Check sheet for the drawn part. Datum: minimum x, y, z corner. Units: mm. Round coordinates to 2 decimals unless told otherwise and drop trailing zeros. Write each loop counter-clockwise with the first axis right and the second up, starting at its lowest first coordinate (ties: lowest second). Pieces come first, ordered by that corner, then holes. Notation, with made-up numbers: (74, 37) -> (103, 37) arc R20 cw to (103, 44) -> close; hole circle Ø4 at (26, -25.5). An arc over 180 degrees is marked (long way). One line per item, written item: value.
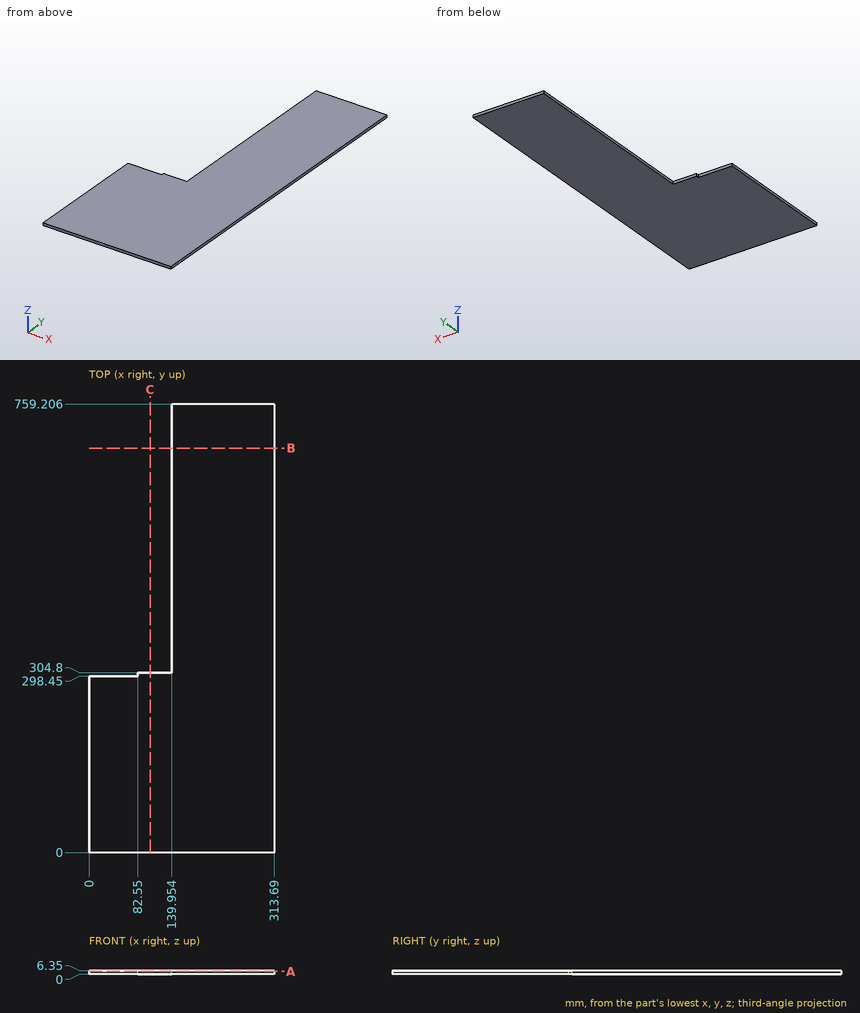
Item 1: Sectioned sample at A-A on z = 5. Enter the section's corners in (x, y).
Answer:
outline: (0, 0) -> (313.69, 0) -> (313.69, 759.21) -> (139.95, 759.21) -> (139.95, 304.8) -> (82.55, 304.8) -> (82.55, 298.45) -> (0, 298.45) -> close
Item 2: Thickness scan on line 1 (Y direction, x = 110, z = 1.75); line 2 (X direction, y = 433.5, z = 4); line 3 (Y direction, x = 17, z = 4.5). Record the ranges inside material, lowest first.
Answer:
line 1: y = 0 to 304.8
line 2: x = 139.95 to 313.69
line 3: y = 0 to 298.45
Item 3: Depth check by flat-ended pin: P1, Ø3, axis at x = 39, z = 4, coming from the +Y side; P2, Ø1.9, axis at x = 100.5, z = 3.5, coming from the +Y side; P3, Ø1.9, axis at y = 645, z = 3, coming from the -X side. Enter the tip coordinate at first touch or a pass-through.
Answer:
P1: stops at y = 298.45
P2: stops at y = 304.8
P3: stops at x = 139.95
Item 4: Sectioned sample at B-B on y = 684.5. Enter the section's corners in (x, z).
Answer:
outline: (139.95, 0) -> (313.69, 0) -> (313.69, 6.35) -> (139.95, 6.35) -> close
Item 5: Sectioned sample at C-C on x = 103.5. Enter the section's corners in (y, z), and give its area (3 significant figures).
Answer:
outline: (0, 0) -> (304.8, 0) -> (304.8, 6.35) -> (0, 6.35) -> close
area: 1,940 mm^2
